Read the model definition and answer for the solid it produces. Units are mm, in the model's axes. Face numbers are marked on the shaded views. Coordinates: 2 decimals unless noted, no trailing zeros. Order: outer loops, then holes, each group sorted by start corner. A loop starts at its lowest first (then second) coordinate and runs counter-clockwise, first axis right, second up. Notation, with made-up numbers: (-8, 8.5) - (50, 8.5) arc R29 cw to (50, 34.5) - close; hole circle Ø10 at (-8.5, 68). An arc over 180 degrees is marked (long way). Use one line per item in the form item = value. Start each with the question number.
from build123d import *

# Parameters (mm, degrees)
F1_DEPTH = 5
F2_DEPTH = 2


with BuildPart() as f1:
    # F0 (on Top) → F1 (new body)
    with BuildSketch(Plane.XY):
        with BuildLine():
            ThreePointArc((-22.322925, 39.647661), (0, 45.5), (22.322925, 39.647661))
            ThreePointArc((22.322925, 39.647661), (26.96297, 46.16557), (21, 51.5))
            Line((21, 51.5), (-21, 51.5))
            ThreePointArc((-21, 51.5), (-26.96297, 46.16557), (-22.322925, 39.647661))
        make_face()
    extrude(amount=F1_DEPTH)

    # F0 (on Top) → F2 (join)
    with BuildSketch(Plane.XY):
        with BuildLine():
            ThreePointArc((21, 39.5), (21.66557, 39.53703), (22.322925, 39.647661))
            ThreePointArc((22.322925, 39.647661), (0, 45.5), (-22.322925, 39.647661))
            ThreePointArc((-22.322925, 39.647661), (-21.66557, 39.53703), (-21, 39.5))
            Line((-21, 39.5), (-21, 32.5))
            Line((-21, 32.5), (21, 32.5))
            Line((21, 32.5), (21, 39.5))
        make_face()
    extrude(amount=F2_DEPTH)


solid = f1.part
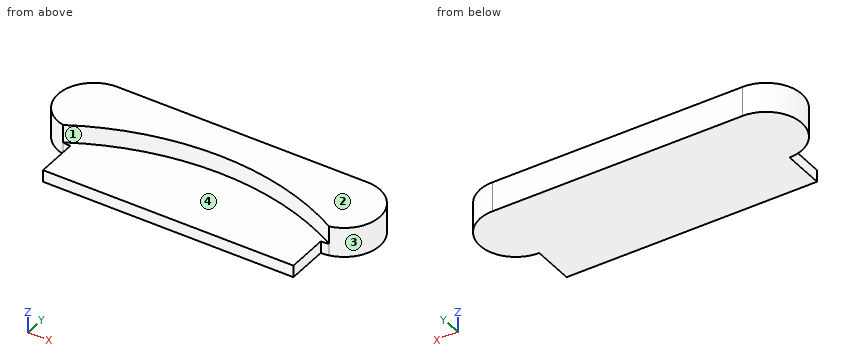
Q1. For a pull along X with two mould halves and no side action, classify the marked faces 1, 2, 3 and 4 as +X half, -X half, draft (parallel to the pull), parting line (faces both ways), or undercut.
Q2. A cutting plane is placed at B-B (z = 3.5). Give the vertices of the cut face in (x, y).
Q3. Given P1, Ø1.5, axis at x = 8, y = 36.5, coming from the +Z side; P2, Ø1, axis at y = 49, z = 3, coming from the -X side; P3, Ø2, axis at y = 36, z = 0.5, coming from the -X side; P4, Ø10, axis at x = -10.5, y = 49, coming from the -Z side, each flat-ended and moving along its own axis, determine where each tip first touches the part or whether it passes through.
Q4. Consider probe 1 along Z at (x, y) = (-14, 34.75); probe 2 along X at (y, z) = (37, 0.4); probe 3 along Y at (x, z) = (10, 4.8). Determine where each line is inside the solid, lowest interval first.
Q5. A cutting plane is placed at A-A (y = 39). Give the vertices of the cut face in (x, z), then the cut area to 3 significant figures.
Q6. A cutting plane is placed at C-C (x = -8). Give the vertices of the cut face in (y, z), then the cut area to 3 significant figures.
Q7. A cutting plane is placed at D-D (y = 42.5). Give the vertices of the cut face in (x, z), then the cut area to 3 significant figures.
Result sheet:
q1.face_1 = undercut
q1.face_2 = draft
q1.face_3 = +X half
q1.face_4 = undercut
q2.outline = (-22.32, 39.65) arc R45.5 cw to (22.32, 39.65) arc R6 ccw to (21, 51.5) - (-21, 51.5) arc R6 ccw to start
q3.P1 = 2
q3.P2 = -26.2
q3.P3 = -21
q3.P4 = 0
q4.probe_1 = 0 to 2
q4.probe_2 = -21 to 21
q4.probe_3 = 44.39 to 51.5
q5.outline = (-21, 0) - (21, 0) - (21, 2) - (-21, 2) - close
q5.area = 84.0 mm^2
q6.outline = (32.5, 0) - (51.5, 0) - (51.5, 5) - (44.79, 5) - (44.79, 2) - (32.5, 2) - close
q6.area = 58.1 mm^2
q7.outline = (-26.2, 0) - (26.2, 0) - (26.2, 5) - (16.25, 5) - (16.25, 2) - (-16.25, 2) - (-16.25, 5) - (-26.2, 5) - close
q7.area = 164 mm^2
